```python
from build123d import *

# Parameters (mm, degrees)
SKETCH_1_R      = 1.4
SKETCH_1_R_2    = 2.266666667
EXTRUDE_1_DEPTH = 193.8


with BuildPart() as part:
    # 草图1 → 凸台-拉伸1 (new body)
    with BuildSketch(Plane.XY):
        with BuildLine():
            Line((5, 23.666666667), (5, 17.866666667))
            ThreePointArc((5, 17.866666667), (5.058578644, 17.72524531), (5.2, 17.666666667))
            Line((5.2, 17.666666667), (6.333333333, 17.666666667))
            Line((6.333333333, 17.666666667), (6.333333333, 20.5))
            Line((6.333333333, 20.5), (8.557190958, 20.5))
            Line((8.557190958, 20.5), (11, 18.057190958))
            Line((11, 18.057190958), (11, 15.346410162))
            Line((11, 15.346410162), (11.199999976, 15.000000042))
            Line((11.199999976, 15.000000042), (11, 14.653589838))
            Line((11, 14.653589838), (11, 11.942809042))
            Line((11, 11.942809042), (8.557190958, 9.5))
            Line((8.557190958, 9.5), (6.333333333, 9.5))
            Line((6.333333333, 9.5), (6.333333333, 12.333333333))
            Line((6.333333333, 12.333333333), (5.2, 12.333333333))
            ThreePointArc((5.2, 12.333333333), (5.058578644, 12.27475469), (5, 12.133333333))
            Line((5, 12.133333333), (5, 6.333333333))
            ThreePointArc((5, 6.333333333), (5.390524292, 5.390524292), (6.333333333, 5))
            Line((6.333333333, 5), (12.133333333, 5))
            ThreePointArc((12.133333333, 5), (12.27475469, 5.058578644), (12.333333333, 5.2))
            Line((12.333333333, 5.2), (12.333333333, 6.333333333))
            Line((12.333333333, 6.333333333), (9.5, 6.333333333))
            Line((9.5, 6.333333333), (9.5, 8.557190958))
            Line((9.5, 8.557190958), (11.942809042, 11))
            Line((11.942809042, 11), (14.653589838, 11))
            Line((14.653589838, 11), (14.999999928, 11.199999958))
            Line((14.999999928, 11.199999958), (15.346410162, 11))
            Line((15.346410162, 11), (18.057190958, 11))
            Line((18.057190958, 11), (20.5, 8.557190958))
            Line((20.5, 8.557190958), (20.5, 6.333333333))
            Line((20.5, 6.333333333), (17.666666667, 6.333333333))
            Line((17.666666667, 6.333333333), (17.666666667, 5.2))
            ThreePointArc((17.666666667, 5.2), (17.72524531, 5.058578644), (17.866666667, 5))
            Line((17.866666667, 5), (23.666666667, 5))
            ThreePointArc((23.666666667, 5), (24.609475708, 5.390524292), (25, 6.333333333))
            Line((25, 6.333333333), (25, 12.133333333))
            ThreePointArc((25, 12.133333333), (24.941421356, 12.27475469), (24.8, 12.333333333))
            Line((24.8, 12.333333333), (23.666666667, 12.333333333))
            Line((23.666666667, 12.333333333), (23.666666667, 9.5))
            Line((23.666666667, 9.5), (21.442809042, 9.5))
            Line((21.442809042, 9.5), (19, 11.942809042))
            Line((19, 11.942809042), (19, 14.653589838))
            Line((19, 14.653589838), (18.800000024, 14.999999958))
            Line((18.800000024, 14.999999958), (19, 15.346410162))
            Line((19, 15.346410162), (19, 18.057190958))
            Line((19, 18.057190958), (21.442809042, 20.5))
            Line((21.442809042, 20.5), (23.666666667, 20.5))
            Line((23.666666667, 20.5), (23.666666667, 17.666666667))
            Line((23.666666667, 17.666666667), (24.8, 17.666666667))
            ThreePointArc((24.8, 17.666666667), (24.941421356, 17.72524531), (25, 17.866666667))
            Line((25, 17.866666667), (25, 23.666666667))
            ThreePointArc((25, 23.666666667), (24.609475708, 24.609475708), (23.666666667, 25))
            Line((23.666666667, 25), (17.866666667, 25))
            ThreePointArc((17.866666667, 25), (17.72524531, 24.941421356), (17.666666667, 24.8))
            Line((17.666666667, 24.8), (17.666666667, 23.666666667))
            Line((17.666666667, 23.666666667), (20.5, 23.666666667))
            Line((20.5, 23.666666667), (20.5, 21.442809042))
            Line((20.5, 21.442809042), (18.057190958, 19))
            Line((18.057190958, 19), (15.346410162, 19))
            Line((15.346410162, 19), (15.000000072, 18.800000042))
            Line((15.000000072, 18.800000042), (14.653589838, 19))
            Line((14.653589838, 19), (11.942809042, 19))
            Line((11.942809042, 19), (9.5, 21.442809042))
            Line((9.5, 21.442809042), (9.5, 23.666666667))
            Line((9.5, 23.666666667), (12.333333333, 23.666666667))
            Line((12.333333333, 23.666666667), (12.333333333, 24.8))
            ThreePointArc((12.333333333, 24.8), (12.27475469, 24.941421356), (12.133333333, 25))
            Line((12.133333333, 25), (6.333333333, 25))
            ThreePointArc((6.333333333, 25), (5.390524292, 24.609475708), (5, 23.666666667))
        make_face()
        with Locations((7.25, 22.75)):
            Circle(SKETCH_1_R, mode=Mode.SUBTRACT)
        with Locations((22.75, 22.75)):
            Circle(SKETCH_1_R, mode=Mode.SUBTRACT)
        with Locations((15, 15)):
            Circle(SKETCH_1_R_2, mode=Mode.SUBTRACT)
        with Locations((7.25, 7.25)):
            Circle(SKETCH_1_R, mode=Mode.SUBTRACT)
        with Locations((22.75, 7.25)):
            Circle(SKETCH_1_R, mode=Mode.SUBTRACT)
    extrude(amount=EXTRUDE_1_DEPTH)


solid = part.part
```
Build history of the part. All positions in model axes, mm. Give positions to 0.01 mm unless a question says otherwise; leave off trailing zeros.
Item 1: Drill centre lines: line 1 (Y direction, x = 7.25, z = 135.5); line 2 (X direction, y = 17.75, z = 16). Where is each one in solid material? Low to high.
Answers follow:
line 1: y = 5 to 5.85, 8.65 to 9.5, 20.5 to 21.35, 24.15 to 25
line 2: x = 5.04 to 6.33, 11 to 19, 23.67 to 24.96
Item 2: Flat gauge pins, fed straight in: pin 1 (1.7 mm diameter, centred on x = 22.75, y = 7.25, fed in from +Z); pin 2 (0.8 mm diameter, centred on y = 13, z = 51, fed in from +X); pin 3 (1.4 mm diameter, centred on x = 14, z = 65.5, fed in from -Y); pin 4 (1.4 mm diameter, centred on y = 16.5, z = 62, fed in from -X). Where does each tip first touch, or does it go through?
Answers follow:
pin 1: passes through
pin 2: stops at x = 19
pin 3: stops at y = 11
pin 4: stops at x = 11
Item 3: Pull direction Y, two halves, no side cores. Call faces 1 (the face through (9, 25, 96)), 2 (the face through (12.736, 15.1, 95.543)), 3 (the face through (25, 21, 96)): released by +Y, released by -Y, zero draft, split by the parting line, or undercut.
Answers follow:
face 1: released by +Y
face 2: undercut
face 3: zero draft
Item 4: Slice it at A-A, the plane z = 182. Give the number of separate pieces and of enclosed holes in the cut face, and give its area (3 significant figures).
Answers follow:
separate pieces: 1
enclosed holes: 5
area: 147 mm2
